from build123d import *

# Parameters (mm, degrees)
SKETCH1_W           = 60
SKETCH1_H           = 50
BOSS_EXTRUDE1_DEPTH = 3
SKETCH2_W           = 20
SKETCH2_H           = 20
CUT_EXTRUDE1_DEPTH  = 3
SKETCH5_R           = 22.5
CUT_EXTRUDE2_DEPTH  = 3
FILLET1_DEPTH       = 3
FILLET1_2_DEPTH     = 3
FILLET2_R           = 2


with BuildPart() as part:
    # Sketch1 → Boss-Extrude1 (new body)
    with BuildSketch(Plane(origin=(0, 0, 0), x_dir=(0, 0, -1), z_dir=(1, 0, 0))):
        with Locations((30, 25)):
            Rectangle(SKETCH1_W, SKETCH1_H)
    extrude(amount=BOSS_EXTRUDE1_DEPTH)

    # Sketch2 → Cut-Extrude1 (cut)
    with BuildSketch(Plane(origin=(3, 0, 0), x_dir=(0, 0, -1), z_dir=(1, 0, 0))):
        with Locations((10, 10)):
            Rectangle(SKETCH2_W, SKETCH2_H)
        with Locations((50, 10)):
            Rectangle(SKETCH2_W, SKETCH2_H)
    extrude(amount=-CUT_EXTRUDE1_DEPTH, mode=Mode.SUBTRACT)

    # Sketch5 → Cut-Extrude2 (cut)
    with BuildSketch(Plane(origin=(3, 0, 0), x_dir=(0, 0, -1), z_dir=(1, 0, 0))):
        with Locations((30, 50)):
            Circle(SKETCH5_R)
    extrude(amount=-CUT_EXTRUDE2_DEPTH, mode=Mode.SUBTRACT)

    # Fillet1: read off the stored shape, not the designer's step
    # Fillet1 outline → Fillet1 (cut)
    with BuildSketch(Plane.YZ):
        with BuildLine():
            ThreePointArc((30, -60), (22.928932188, -57.071067812), (20, -50))
            Line((20, -50), (20, -60))
            Line((20, -60), (30, -60))
        make_face()
        with BuildLine():
            ThreePointArc((20, -10), (22.928932188, -2.928932188), (30, 0))
            Line((30, 0), (20, 0))
            Line((20, 0), (20, -10))
        make_face()
    extrude(amount=FILLET1_DEPTH, mode=Mode.SUBTRACT)

    # Fillet1 2 outline → Fillet1 2 (add)
    with BuildSketch(Plane.YZ):
        with BuildLine():
            ThreePointArc((10, -40), (17.071067812, -42.928932188), (20, -50))
            Line((20, -50), (20, -40))
            Line((20, -40), (10, -40))
        make_face()
        with BuildLine():
            Line((20, -20), (20, -10))
            ThreePointArc((20, -10), (17.071067812, -17.071067812), (10, -20))
            Line((10, -20), (20, -20))
        make_face()
    extrude(amount=FILLET1_2_DEPTH)

    # Fillet2
    fillet2_edges = [part.edges().sort_by_distance(p)[0] for p in [
        (1.5, 50, -52.5),
        (1.5, 50, -7.5),
        (1.5, 50, 0),
        (1.5, 50, -60),
    ]]
    fillet(fillet2_edges, radius=FILLET2_R)


solid = part.part
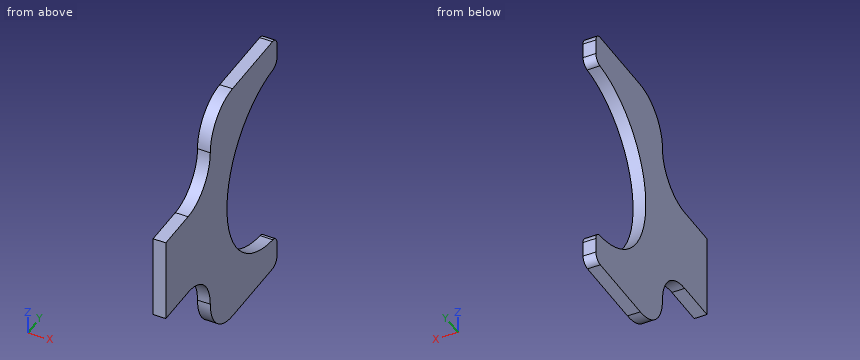
The listing builds one solid part. Answer for the finished solid, in the listing's coordinates (mm). Round coordinates to 2 decimals unless told otherwise and drop trailing zeros. Order: outer loops, then holes, each group sorted by start corner. A loop starts at its lowest first (then second) coordinate and runs counter-clockwise, first axis right, second up. Notation, with made-up numbers: M 7,27 L 44,27 A20 cw 44,64 Z; hole C 68.5,40 d3. An arc over 180 degrees is marked long. Answer in a Markdown table with one row per item. Add a question column.
1) Flat-ended cylindrical pins translate along their axes: pin 1 Ø1.5 at (x, z) = (1, -16.5) entering from +Y; pin 2 Ø1.5 at (x, y) = (1, 6.5) entering from -Z; pin 3 Ø1 at (x, y) = (2.5, 29) entering from -Z. Find the tip coordinate at first contact, or state that the pin passes through.
2) The part is cut by section C-C on z = -4. Determine the outline of the cut face in (x, y), plus the area to 3 significant figures.
3) Consider line 1 along Z through (x, y) = (2.05, 5.5); line 2 along Z through (x, y) = (2.75, 37); line 3 along Z through (x, y) = (0.95, 42). Determine where each line is inside the solid, lowest interval first. Write a range as from..to.
4) The part is cut by section B-B on x = 1.75. Determine the outline of the cut face in (y, z), plus the area to 3 significant figures.
5) The part is cut by section A-A on y = 45. Determine the outline of the cut face in (x, z), plus the area to 3 significant figures.
6) The part is cut by section D-D on y = 31. Determine the outline of the cut face in (x, z), plus the area to 3 significant figures.
Findings below:
| question | item | result |
|---|---|---|
| 1 | pin 1 | stops at y = 32.59 |
| 1 | pin 2 | stops at z = -40 |
| 1 | pin 3 | stops at z = -59.99 |
| 2 | outline | M 0,22 L 3,22 L 3,50 L 0,50 Z |
| 2 | area | 84.0 mm² |
| 3 | line 1 | z = -40..-20 |
| 3 | line 2 | z = -60..-48.36, -11.64..0 |
| 3 | line 3 | z = -60..-51.03, -8.97..0 |
| 4 | outline | M 0,-40 L 10,-40 A10 cw 20,-50 A10 ccw 30,-60 L 48,-60 A2 ccw 50,-58 L 50,-54.42 A2 ccw 48.16,-52.42 A22.5 cw 48.16,-7.58 A2 ccw 50,-5.58 L 50,-2 A2 ccw 48,0 L 30,0 A10 ccw 20,-10 A10 cw 10,-20 L 0,-20 Z |
| 4 | area | 1,400 mm² |
| 5 | outline | M 0,-60 L 3,-60 L 3,-51.94 L 0,-51.94 Z; M 0,-8.06 L 3,-8.06 L 3,0 L 0,0 Z |
| 5 | area | 48.4 mm² |
| 6 | outline | M 0,-60 L 3,-60 L 3,-42.05 L 0,-42.05 Z; M 0,-17.95 L 3,-17.95 L 3,0 L 0,0 Z |
| 6 | area | 108 mm² |
